```python
from build123d import *

# Parameters (mm, degrees)
EXTRUDE1_DEPTH = 10


with BuildPart() as part:
    # Sketch1 → Extrude1 (new body)
    with BuildSketch(Plane.XY):
        with BuildLine():
            Line((-4.285898385, 0), (4.285898385, 0))
            ThreePointArc((4.285898385, 0), (5.285898385, -0.267949192), (6.017949192, -1))
            ThreePointArc((6.017949192, -1), (8.26763809, -1.931851653), (9.75, 0))
            Line((9.75, 0), (9.75, 32))
            ThreePointArc((9.75, 32), (10.042893219, 32.707106781), (10.75, 33))
            Line((10.75, 33), (21.5, 33))
            ThreePointArc((21.5, 33), (21.853553391, 33.146446609), (22, 33.5))
            Line((22, 33.5), (22, 39))
            ThreePointArc((22, 39), (21.853553391, 39.353553391), (21.5, 39.5))
            Line((21.5, 39.5), (15.5, 39.5))
            ThreePointArc((15.5, 39.5), (15.146446609, 39.646446609), (15, 40))
            Line((15, 40), (15, 46))
            ThreePointArc((15, 46), (15.146446609, 46.353553391), (15.5, 46.5))
            Line((15.5, 46.5), (22.5, 46.5))
            ThreePointArc((22.5, 46.5), (22.853553391, 46.646446609), (23, 47))
            Line((23, 47), (23, 47.5))
            ThreePointArc((23, 47.5), (23.146446609, 47.853553391), (23.5, 48))
            Line((23.5, 48), (28.286569779, 48))
            ThreePointArc((28.286569779, 48), (30.671448312, 47.39458239), (32.478787861, 45.724941753))
            Line((32.478787861, 45.724941753), (36.692218082, 39.242741413))
            ThreePointArc((36.692218082, 39.242741413), (37.293802791, 37.938874885), (37.5, 36.51779966))
            Line((37.5, 36.51779966), (37.5, -17.210914823))
            ThreePointArc((37.5, -17.210914823), (38.56139741, -23.639704129), (41.632933194, -29.386143403))
            Line((41.632933194, -29.386143403), (166.933533403, -192.681064827))
            ThreePointArc((166.933533403, -192.681064827), (168.469301295, -195.554284464), (169, -198.768679117))
            Line((169, -198.768679117), (169, -220.5))
            ThreePointArc((169, -220.5), (168.121320344, -222.621320344), (166, -223.5))
            Line((166, -223.5), (92, -223.5))
            ThreePointArc((92, -223.5), (89.878679656, -222.621320344), (89, -220.5))
            Line((89, -220.5), (89, -195.799020434))
            ThreePointArc((89, -195.799020434), (88.537169507, -192.791962439), (87.191520443, -190.06325607))
            Line((87.191520443, -190.06325607), (-14.488629988, -44.848951908))
            ThreePointArc((-14.488629988, -44.848951908), (-15.609082619, -43.513648459), (-16.944386067, -42.393195828))
            Line((-16.944386067, -42.393195828), (-24.707293091, -36.957549812))
            ThreePointArc((-24.707293091, -36.957549812), (-34.110324995, -26.23544688), (-37.5, -12.382988483))
            Line((-37.5, -12.382988483), (-37.5, 36.51779966))
            ThreePointArc((-37.5, 36.51779966), (-37.293802791, 37.938874885), (-36.692218082, 39.242741413))
            Line((-36.692218082, 39.242741413), (-32.478787861, 45.724941753))
            ThreePointArc((-32.478787861, 45.724941753), (-30.671448312, 47.39458239), (-28.286569779, 48))
            Line((-28.286569779, 48), (-23.5, 48))
            ThreePointArc((-23.5, 48), (-23.146446609, 47.853553391), (-23, 47.5))
            Line((-23, 47.5), (-23, 47))
            ThreePointArc((-23, 47), (-22.853553391, 46.646446609), (-22.5, 46.5))
            Line((-22.5, 46.5), (-15.5, 46.5))
            ThreePointArc((-15.5, 46.5), (-15.146446609, 46.353553391), (-15, 46))
            Line((-15, 46), (-15, 40))
            ThreePointArc((-15, 40), (-15.146446609, 39.646446609), (-15.5, 39.5))
            Line((-15.5, 39.5), (-21.5, 39.5))
            ThreePointArc((-21.5, 39.5), (-21.853553391, 39.353553391), (-22, 39))
            Line((-22, 39), (-22, 33.5))
            ThreePointArc((-22, 33.5), (-21.853553391, 33.146446609), (-21.5, 33))
            Line((-21.5, 33), (-10.75, 33))
            ThreePointArc((-10.75, 33), (-10.042893219, 32.707106781), (-9.75, 32))
            Line((-9.75, 32), (-9.75, 0))
            ThreePointArc((-9.75, 0), (-8.26763809, -1.931851653), (-6.017949192, -1))
            ThreePointArc((-6.017949192, -1), (-5.285898385, -0.267949192), (-4.285898385, 0))
        make_face()
    extrude(amount=EXTRUDE1_DEPTH)


solid = part.part
```
Input: part model. Units: mm. Frame: model coordinates. A direction names the side the tool comes from. Give positions to 0.01 mm unless a question says otherwise; leave off trailing zeros. Write each loop counter-clockwise with the first axis right and the second up, starting at its lowest first coordinate (ties: lowest second). Pieces come first, ordered by that corner, then holes. Notation, with made-up numbers: (27, 0.5) - (33, 0.5) arc R24 ccw to (33, 39.5) - close; hole circle Ø11 at (24.25, 30). An arc over 180 degrees is marked (long way). Write item = value, one per line. Start each with the question number.
1) Cut plane A-A (x = 97). Return loops of the section in (y, z), and give its area (3 significant figures).
2) Reachability of faces 4 (the face through (22, 36, 5)), 5 (the face through (130, -223.5, 5)), 6 (the face through (37.5, 10, 5)), 7 (the face through (-19, 46.5, 5)) from +Z, -Z, +X, -X, +Y, -Y: full face, straight path, thin tool, end or side. Return the list, or none.
3) Material intervals for L1, parallel to X at y = 16.5, z = 5.25; L2, parallel to X at y = -200.5, z = 4.75; L3, parallel to X at y = -4.5, z = 9, sorted ascending. Write a range as [from, to].
4) Pin query (flat end, axial travel): pin 1 (3 mm diameter, centred on x = 15, z = 4.5, fed in from +Y); pin 2 (5 mm diameter, centred on x = 110.5, z = 5.5, fed in from +Y); pin 3 (1 mm diameter, centred on y = -50.5, z = 6, fed in from +X). Return the tip coordinate at first contact, or that it passes through.
5) Cut plane B-B (y = -175). Return loops of the section in (x, z), and give its area (3 significant figures).
6) Draft query along Y for faces 1 (the face through (16, 33, 5)), 2 (the face through (-34.02, -26.41, 4.93)), 3 (the face through (51, -97, 0)). Return one class per face: pulls with the +Y half, pulls with the -Y half, needs draft (parallel to the pull), parting line crosses it, or undercut.
Answers follow:
q1.outline = (-223.5, 0) - (-101.54, 0) - (-101.54, 10) - (-223.5, 10) - close
q1.area = 1,220 mm^2
q2.face_4 = +Z, -Z
q2.face_5 = +Z, -Z, +X, -X, -Y
q2.face_6 = +Z, -Z, +X, +Y
q2.face_7 = +Z, -Z, +Y
q3.L1 = [-37.5, -9.75], [9.75, 37.5]
q3.L2 = [89, 169]
q3.L3 = [-37.5, 37.5]
q4.pin_1 = 46.5
q4.pin_2 = -115.88
q4.pin_3 = 58.22
q5.outline = (76.64, 0) - (153.37, 0) - (153.37, 10) - (76.64, 10) - close
q5.area = 767 mm^2
q6.face_1 = undercut
q6.face_2 = pulls with the -Y half
q6.face_3 = needs draft
